```python
from build123d import *

# Parameters (mm, degrees)
F0_R     = 57.15
F1_DEPTH = 6.35


with BuildPart() as f1:
    # F0 (on Top) → F1 (new body)
    with BuildSketch(Plane.XY):
        with BuildLine():
            Line((50.401562, 196.85), (-50.401562, 196.85))
            ThreePointArc((-50.401562, 196.85), (-76.714053, 188.16268), (-101.6, 175.976362))
            ThreePointArc((-101.6, 175.976362), (-124.596634, 160.517659), (-145.276319, 142.074033))
            Line((-145.276319, 142.074033), (-195.677882, 54.775967))
            ThreePointArc((-195.677882, 54.775967), (-203.2, 0), (-195.677882, -54.775967))
            Line((-195.677882, -54.775967), (-145.276319, -142.074033))
            ThreePointArc((-145.276319, -142.074033), (-101.6, -175.976362), (-50.401562, -196.85))
            Line((-50.401562, -196.85), (50.401562, -196.85))
            ThreePointArc((50.401562, -196.85), (101.6, -175.976362), (145.276319, -142.074033))
            Line((145.276319, -142.074033), (195.677882, -54.775967))
            ThreePointArc((195.677882, -54.775967), (203.2, 0), (195.677882, 54.775967))
            Line((195.677882, 54.775967), (145.276319, 142.074033))
            ThreePointArc((145.276319, 142.074033), (101.6, 175.976362), (50.401562, 196.85))
        make_face()
        with Locations((-61.9125, -107.235596)):
            Circle(F0_R, mode=Mode.SUBTRACT)
        with Locations((61.9125, -107.235596)):
            Circle(F0_R, mode=Mode.SUBTRACT)
        with Locations((-123.825, 0)):
            Circle(F0_R, mode=Mode.SUBTRACT)
        with BuildLine():
            ThreePointArc((6.35, 0), (-3.175, -5.499261), (-3.175, 5.499261))
            ThreePointArc((-3.175, 5.499261), (3.175, 5.499261), (6.35, 0))
        make_face(mode=Mode.SUBTRACT)
        with BuildLine():
            ThreePointArc((-33.3375, 57.742244), (-111.405852, 78.660596), (-90.4875, 156.728947))
            ThreePointArc((-90.4875, 156.728947), (-33.3375, 156.728947), (-4.7625, 107.235596))
            ThreePointArc((-4.7625, 107.235596), (-12.419148, 78.660596), (-33.3375, 57.742244))
        make_face(mode=Mode.SUBTRACT)
        with Locations((123.825, 0)):
            Circle(F0_R, mode=Mode.SUBTRACT)
        with Locations((61.9125, 107.235596)):
            Circle(F0_R, mode=Mode.SUBTRACT)
    extrude(amount=F1_DEPTH)


solid = f1.part
```
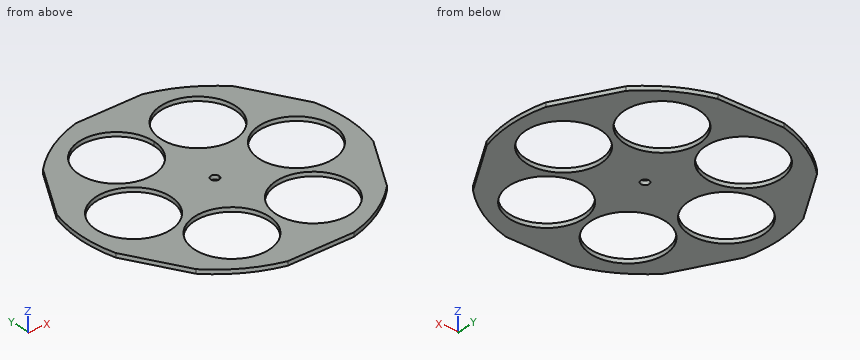
Can you work these out from the model? Positions are in its coordinate system, mm. Give positions to 0.01 mm unless a question says otherwise; leave off trailing zeros. Order: outer loops, then holes, each group sorted by start corner. A loop starts at its lowest first (then second) coordinate and runs counter-clockwise, first axis right, second up. Notation, with made-up numbers: M 51,4.25 L 63,4.25 A29 cw 63,42.25 Z; hole C 21,-9 d1. An arc over 180 degrees is marked long. Write item = value, one per line. Start each with the question number.
Q1. Suppose I cut it at B-B (x = -74). Write out the boundary of the cut face in (y, z).
Q2. Suppose I cut it at D-D (x = -134.5). Write out the boundary of the cut face in (y, z).
Q3. I need wall thicknesses on probe 1 along Y at (x, z) = (0, 4); probe 2 along Y at (x, z) = (-27, 2); probe 3 along Y at (x, z) = (-32, 1.75). Which ranges of each line are inside material? Lowest first, please. Write a range as [from, to].
Q4. Suppose I cut it at A-A (y = 29). Write out the boundary of the cut face in (x, z), plus the area to 3 significant figures.
Q5. Suppose I cut it at C-C (z = 1.5). Count the separate pieces of the cut face and the enclosed holes in it, plus the area to 3 significant figures.
Check result:
q1.outline = M -189.25,0 L -163.09,0 L -163.09,6.35 L -189.25,6.35 Z; M -51.38,0 L -27.99,0 L -27.99,6.35 L -51.38,6.35 Z; M 27.99,0 L 51.38,0 L 51.38,6.35 L 27.99,6.35 Z; M 163.09,0 L 189.25,0 L 189.25,6.35 L 163.09,6.35 Z
q2.outline = M -152.32,0 L -56.14,0 L -56.14,6.35 L -152.32,6.35 Z; M 56.14,0 L 152.32,0 L 152.32,6.35 L 56.14,6.35 Z
q3.probe_1 = [-196.85, -6.35], [6.35, 196.85]
q3.probe_2 = [-196.85, -152.48], [-61.99, 61.99], [152.48, 196.85]
q3.probe_3 = [-196.85, -155.93], [-58.54, 58.54], [155.93, 196.85]
q4.outline = M -201.12,0 L -173.07,0 L -173.07,6.35 L -201.12,6.35 Z; M -74.58,0 L 74.58,0 L 74.58,6.35 L -74.58,6.35 Z; M 173.07,0 L 201.12,0 L 201.12,6.35 L 173.07,6.35 Z
q4.area = 1,300 mm2
q5.separate_pieces = 1
q5.enclosed_holes = 7
q5.area = 65,500 mm2
